Source: CAD feature listing. Evaluate the final solid. Frame: model axes, mm. A direction names the side the tool comes from. Coordinates: 2 decimals unless noted, no trailing zeros. Order: outer loops, then holes, each group sorted by start corner. A loop starts at its lowest first (then second) coordinate and runs counter-clockwise, first axis right, second up.
Item 1: Ray query, line 1 (Z direction, x = 13, y = -5); line 2 (Y direction, x = 11.5, z = 1.9); line 3 (Y direction, x = 7, z = 1.65). Return the intervals inside material, ascending.
Item 2: Mould query, pull axis X, two halves, no side actions, for faces 4 (the cylindrical face through (19.144, -0.219, 0.986)), 5 (the flat face through (-12.312, -0.6, 2.5)), 6 (the flat face through (4.2, -6.997, 2.5)), 7 (the flat face through (5.148, -2.863, 0.986)). Classes: released by +X, released by -X, zero draft, split by the parting line, or undercut.
Item 3: Contact query for a flat-ended pin moving along its axis: P1, Ø1, axis at x = 0, y = -1, coming from the -Z side. Output: stop coordinate, or through.
Item 4: Section B-B on y = 0. Return the cut outline in (x, z), then the cut area to 3 significant figures.
Item 5: Reachability of faces 1 (the flat face through (4, 4, 0)), 2 (the cylindrical face through (-10.6, 0.1, 1)), 3 (the flat face through (4.87, 2.88, 0.99)) from +Z, -Z, +X, -X, +Y, -Y: full face, straight path, thin tool, end or side. Return the list, or none.
Item 6: Section D-D on y = 4.75. Return the cut outline in (x, z).
Item 7: Section C-C on x = 18.5. Return the cut outline in (y, z), then the cut area to 3 significant figures.
Item 8: Section A-A on z = 0.6. Return the cut outline in (x, y), then the cut area to 3 significant figures.
from build123d import *

# Parameters (mm, degrees)
BOSS_EXTRUDE1_DEPTH = 2
SKETCH2_W           = 33.530667502
SKETCH2_H           = 12.876796265
BOSS_EXTRUDE2_DEPTH = 1


with BuildPart() as part:
    # Sketch1 → Boss-Extrude1 (new body)
    with BuildSketch(Plane(origin=(0, 0, 0), x_dir=(-1, 0, 0), z_dir=(0, 0, 1))):
        with BuildLine():
            Line((4.419624532, 5.457754962), (-15.163378573, 4.241831176))
            ThreePointArc((-15.163378573, 4.241831176), (-19.147983311, 0.130911389), (-15.424074318, -4.217564002))
            Line((-15.424074318, -4.217564002), (-14.905016784, -4.249997039))
            Line((-14.905016784, -4.249997039), (4.41534389, -5.457219623))
            Line((4.41534389, -5.457219623), (5.1, -5.5))
            ThreePointArc((5.1, -5.5), (10.6, 0), (5.1, 5.5))
            Line((5.1, 5.5), (4.419624532, 5.457754962))
        make_face()
        with BuildLine():
            Line((-14.9, 2.25), (4.880474733, 3.493108738))
            ThreePointArc((4.880474733, 3.493108738), (8.6, 0), (4.880474733, -3.493108738))
            Line((4.880474733, -3.493108738), (-14.9, -2.25))
            ThreePointArc((-14.9, -2.25), (-17.15, 0), (-14.9, 2.25))
        make_face(mode=Mode.SUBTRACT)
    extrude(amount=BOSS_EXTRUDE1_DEPTH)

    # Sketch2 → Boss-Extrude2 (add)
    with BuildSketch(Plane.XY.offset(2)):
        with Locations((4.453710744, -0.558629325)):
            Rectangle(SKETCH2_W, SKETCH2_H)
    extrude(amount=BOSS_EXTRUDE2_DEPTH)


solid = part.part
Answer list:
1. line 1: z = 2 to 3
1. line 2: y = -4.47 to -2.46, 2.46 to 4.46
1. line 3: y = -4.75 to -2.75, 2.75 to 4.74
2. face 4: released by +X
2. face 5: released by -X
2. face 6: zero draft
2. face 7: undercut
3. P1: stops at z = 2
4. outline: (-12.31, 2) - (-10.6, 2) - (-10.6, 0) - (-8.6, 0) - (-8.6, 2) - (17.15, 2) - (17.15, 0) - (19.15, 0) - (19.15, 2) - (21.22, 2) - (21.22, 3) - (-12.31, 3) - close
4. area: 41.5 mm2
5. face 1: -Z, +X, -X, +Y, -Y
5. face 2: -Z, -X
5. face 3: -Z
6. outline: (-12.31, 2) - (-7.87, 2) - (-7.87, 0) - (6.9, 0) - (6.9, 2) - (21.22, 2) - (21.22, 3) - (-12.31, 3) - close
7. outline: (-7, 2) - (-2.26, 2) - (-2.26, 0) - (2.26, 0) - (2.26, 2) - (5.88, 2) - (5.88, 3) - (-7, 3) - close
7. area: 21.9 mm2
8. outline: (-5.1, -5.5) - (15.16, -4.24) arc R4.25 ccw to (15.42, 4.22) - (-5.1, 5.5) arc R5.5 ccw to start; hole (-4.88, -3.49) - (14.9, -2.25) arc R2.25 ccw to (14.9, 2.25) - (-4.88, 3.49) arc R3.5 ccw (long way) to start
8. area: 129 mm2
